Autodesk Inventor part; units mm, degrees
ref_plane "YZ Plane" through (0, 0, 0) normal (1, 0, 0) x (0, 1, 0)
ref_plane "XZ Plane" through (0, 0, 0) normal (0, 1, 0) x (-1, 0, 0)
ref_plane "XY Plane" through (0, 0, 0) normal (0, 0, 1) x (1, 0, 0)
sketch "Sketch1" plane through (0, 0, 0) normal (0, 1, 0) x (-1, 0, 0)
  line L0 (41.275, 330.2) -> (-41.275, 330.2)
  line L1 (-41.275, 330.2) -> (-41.275, -330.2)
  line L2 (-41.275, -330.2) -> (41.275, -330.2)
  line L3 (41.275, -330.2) -> (41.275, 330.2)
  line L4 (41.275, 330.2) -> (-41.275, -330.2) construction
  line L5 (-41.275, 330.2) -> (41.275, -330.2) construction
  point P0 (0, 0)
  dimension "d0" = 82.55
  dimension "d1" = 660.4
extrude "Extrusion1" add sketch "Sketch1" along normal mid plane 1.5875
sketch "Sketch2" plane through (41.275, 0.7937, -330.2) normal (0, 0, -1) x (-1, 0, 0)
  line L0 (90.4875, -7.9375) -> (90.4875, -58.7375)
  line L1 (90.4875, -58.7375) -> (88.9, -58.7375)
  line L2 (88.9, -58.7375) -> (88.9, -7.9375)
  arc A0 (88.9, -7.9375) -> (82.55, -1.5875) centre (82.55, -7.9375) ccw
  line L3 (82.55, -1.5875) -> (82.55, 0)
  arc A1 (90.4875, -7.9375) -> (82.55, 0) centre (82.55, -7.9375) ccw
  point P0 (41.275, -0.7937)
  dimension "d4" = 6.35
  dimension "d5" = 57.15
  dimension "d6" = 1.5875
extrude "Extrusion2" add sketch "Sketch2" against normal blind 660.4
sketch "Sketch3" plane through (-49.2125, -57.9438, -330.2) normal (-1, 0, 0) x (0, 0, 1)
  arc A0 (518.9985, 0) -> (520.5697, 1.8143) centre (518.9985, 1.5875) ccw
  arc A1 (520.5697, 1.8143) -> (508, 12.7) centre (508, 0) ccw
  line L0 (497.2617, 12.7) -> (508, 12.7)
  line L1 (413.9219, 12.7) -> (497.2617, 12.7)
  line L2 (330.2, 12.7) -> (413.9219, 12.7)
  line L3 (226.8601, 12.7) -> (330.2, 12.7)
  line L4 (158.6559, 12.7) -> (226.8601, 12.7)
  line L5 (152.4, 12.7) -> (158.6559, 12.7)
  arc A2 (152.4, 12.7) -> (139.8303, 1.8143) centre (152.4, 0) ccw
  arc A3 (139.8303, 1.8143) -> (141.4015, 0) centre (141.4015, 1.5875) ccw
  line L6 (518.9985, 0) -> (141.4015, 0)
  line L7 (497.2617, 22.225) -> (508, 22.225)
  arc A4 (529.997, 3.175) -> (508, 22.225) centre (508, 0) ccw
  arc A5 (518.9985, -9.525) -> (529.997, 3.175) centre (518.9985, 1.5875) ccw
  line L8 (518.9985, -9.525) -> (141.4015, -9.525)
  arc A6 (130.403, 3.175) -> (141.4015, -9.525) centre (141.4015, 1.5875) ccw
  arc A7 (152.4, 22.225) -> (130.403, 3.175) centre (152.4, 0) ccw
  line L9 (152.4, 22.225) -> (158.6559, 22.225)
  line L10 (158.6559, 22.225) -> (226.8601, 22.225)
  line L11 (226.8601, 22.225) -> (330.2, 22.225)
  line L12 (330.2, 22.225) -> (413.9219, 22.225)
  line L13 (413.9219, 22.225) -> (497.2617, 22.225)
  point P0 (330.2, 57.9438)
  dimension "d9" = 9.525
extrude "Extrusion3" cut sketch "Sketch3" against normal up to surface (1.5875 mm away) contours L6 A3 A2 L5 L4 L3 L2 L1 L0 A1 A0 | L7 A4 A5 L8 A6 A7 L9 L10 L11 L12 L13
sketch "Sketch5" plane through (-49.2125, -57.9438, -330.2) normal (-1, 0, 0) x (0, 0, 1)
  line L0 (515.6192, 11.1235) -> (519.405, 9.6946)
  line L1 (518.9828, 20.0348) -> (522.7587, 18.6096)
  line L2 (518.9828, 20.0348) -> (513.1799, 22.225)
  line L3 (513.1799, 22.225) -> (508, 22.225)
  arc A0 (529.997, 3.175) -> (508, 22.225) centre (508, 0) ccw
  line L4 (522.7587, 18.6096) -> (572.0643, 0)
  line L5 (529.997, 0) -> (660.4, 0)
  arc A1 (130.403, 3.175) -> (130.403, 0) centre (141.4015, 1.5875) ccw
  arc A2 (152.4, 22.225) -> (130.403, 3.175) centre (152.4, 0) ccw
  line L6 (152.4, 22.225) -> (508, 22.225)
  arc A3 (529.997, 3.175) -> (508, 22.225) centre (508, 0) ccw
  arc A4 (529.997, 0) -> (529.997, 3.175) centre (518.9985, 1.5875) ccw
  line L7 (529.997, 0) -> (660.4, 0)
  line L8 (660.4, 50.8) -> (660.4, 0)
  line L9 (0, 50.8) -> (660.4, 50.8)
  line L10 (0, 0) -> (0, 50.8)
  line L11 (0, 0) -> (130.403, 0)
  point P0 (330.2, 57.9438)
  dimension "d12" = 9.525
extrude "Extrusion4" cut sketch "Sketch5" against normal up to surface (1.5875 mm away) contours L1 L4 L5 A4 A0 L3 L2
fillet "Fillet1" radius 3.175 2 edges at (-48.4188, -57.9438, -199.797) (-48.4188, -35.7187, 182.9799)
fillet "Fillet2" radius 3.175 4 edges at (-48.4188, -57.9438, -330.2) (41.275, 0, -330.2) (-48.4188, -57.9438, 330.2) (41.275, 0, 330.2)
properties part number "TopPlate" material "ABS Plastic"
CAD build for the part. Positions are in the model's coordinates, mm. A direction names the side the tool comes from. Round coordinates to 2 decimals unless told otherwise and drop trailing zeros. Write each loop counter-clockwise with the first axis right and the second up, starting at its lowest first coordinate (ties: lowest second). Pieces come first, ordered by that corner, then holes. Notation, with made-up numbers: M -3,48.5 L 40,48.5 A27 cw 40,69.5 Z; hole C -36,81.25 d10. An arc over 180 degrees is marked long. Use a Markdown table: item, result. Add a question column.
1. Flat gauge pins, fed straight in: P1, Ø1, axis at y = -25.5, z = -219.5, coming from the +X side (3 decimals); P2, Ø25, axis at x = -11.5, z = -84.5, coming from the -Y side; P3, Ø0.5, axis at x = -48.5, z = -49, coming from the -Y side. Where does each tip first touch, or does it go through?
2. 3-axis set-ups, long thin cutter, end or side, ignore diameter. For faces 4 (the face through (-5, 0, 330.2)), 5 (the face through (1, -0.794, 5)): which of +Z, -Z, +X, -X, +Y, -Y reach the whole face in a straight line?
3. Pull direction Z, two halves, no side cores. Call faces 1 (the face through (-48.43, -41, -192.18)), 2 (the face through (-5, 0, -330.2)), 3 (the face through (-47.625, -27, -5)): released by +Z, released by -Z, zero draft, split by the parting line, or undercut.
4. Drill centre lines: probe 1 along X at (y, z) = (-27.5, 13.5) (1 decimal); probe 2 along Y at (x, z) = (19, 115.5); probe 3 along Y at (x, z) = (-44, -221). Where is each one in solid material? Low to high.
5. Slice it at D-D on x = 28. Give the cut face in (y, z), then the cut area to 3 significant figures.
6. Slice it at B-B on y = -48. Give the cut face in (x, z) (1 decimal).
Reply:
| question | item | result |
|---|---|---|
| 1 | P1 | stops at x = -47.625 |
| 1 | P2 | stops at y = -0.79 |
| 1 | P3 | stops at y = -35.72 |
| 2 | face 4 | +Z, +X, -X, +Y, -Y |
| 2 | face 5 | +Z, -Z, +X, -Y |
| 3 | face 1 | undercut |
| 3 | face 2 | released by -Z |
| 3 | face 3 | zero draft |
| 4 | probe 1 | x = -49.2 to -47.6 |
| 4 | probe 2 | y = -0.79 to 0.79 |
| 4 | probe 3 | y = -1.41 to 0.31 |
| 5 | outline | M -0.79,-330.2 L 0.79,-330.2 L 0.79,330.2 L -0.79,330.2 Z |
| 5 | area | 1,050 mm^2 |
| 6 | outline | M -49.2,-330.2 L -47.6,-330.2 L -47.6,-197.7 L -49.2,-197.7 Z; M -49.2,215.5 L -47.6,215.5 L -47.6,330.2 L -49.2,330.2 Z |
